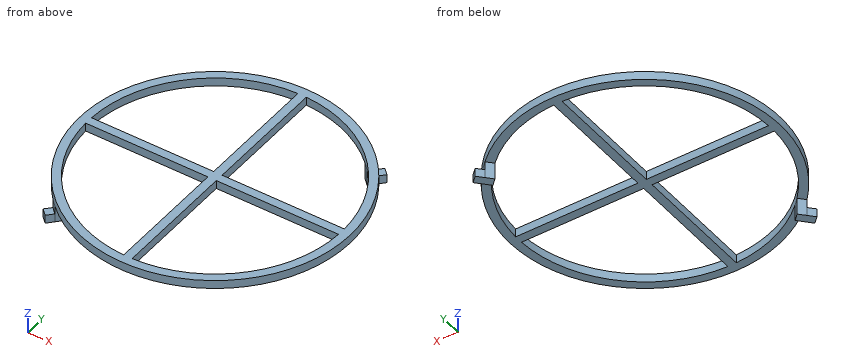
from build123d import *

# Parameters (mm, degrees)
SKETCH1_R           = 16
BOSS_EXTRUDE1_DEPTH = 1
BOSS_EXTRUDE2_DEPTH = 1
BOSS_EXTRUDE3_DEPTH = 1
CIRPATTERN1_COUNT   = 2


with BuildPart() as part:
    # Sketch1 → Boss-Extrude1 (new body)
    with BuildSketch(Plane.XY):
        Circle(SKETCH1_R)
        with BuildLine():
            Line((-0.5, 14.991664351), (-0.5, 0.5))
            Line((-0.5, 0.5), (-14.991664351, 0.5))
            ThreePointArc((-14.991664351, 0.5), (-10.606601718, 10.606601718), (-0.5, 14.991664351))
        make_face(mode=Mode.SUBTRACT)
        with BuildLine():
            Line((0.5, 14.991664351), (0.5, 0.5))
            Line((0.5, 0.5), (14.991664351, 0.5))
            ThreePointArc((14.991664351, 0.5), (10.606601718, 10.606601718), (0.5, 14.991664351))
        make_face(mode=Mode.SUBTRACT)
        with BuildLine():
            Line((-14.991664351, -0.5), (-0.5, -0.5))
            Line((-0.5, -0.5), (-0.5, -14.991664351))
            ThreePointArc((-0.5, -14.991664351), (-10.606601718, -10.606601718), (-14.991664351, -0.5))
        make_face(mode=Mode.SUBTRACT)
        with BuildLine():
            Line((0.5, -0.5), (14.991664351, -0.5))
            ThreePointArc((14.991664351, -0.5), (10.606601718, -10.606601718), (0.5, -14.991664351))
            Line((0.5, -14.991664351), (0.5, -0.5))
        make_face(mode=Mode.SUBTRACT)
    extrude(amount=BOSS_EXTRUDE1_DEPTH)

    # Sketch3 → Boss-Extrude2 (add)
    with BuildSketch(Plane(origin=(0, 0, 0), x_dir=(-1, 0, 0), z_dir=(0, 0, -1))):
        with BuildLine():
            Line((-11.661770518, 10.954593027), (-10.97567443, 10.224214923))
            ThreePointArc((-10.97567443, 10.224214923), (-10.628744174, 10.58441294), (-10.269999326, 10.932845642))
            Line((-10.269999326, 10.932845642), (-10.954665948, 11.661702018))
            ThreePointArc((-10.954665948, 11.661702018), (-11.313743872, 11.313673126), (-11.661770518, 10.954593027))
        make_face()
    boss_extrude2 = extrude(amount=BOSS_EXTRUDE2_DEPTH)

    # Sketch4 → Boss-Extrude3 (add)
    with BuildSketch(Plane(origin=(0, 0, -1), x_dir=(-1, 0, 0), z_dir=(0, 0, -1))):
        with BuildLine():
            Line((-11.661770518, 10.954593027), (-10.97567443, 10.224214923))
            ThreePointArc((-10.97567443, 10.224214923), (-10.628744174, 10.58441294), (-10.269999326, 10.932845642))
            Line((-10.269999326, 10.932845642), (-10.954665948, 11.661702018))
            Line((-10.954665948, 11.661702018), (-11.617936738, 12.367781633))
            Line((-11.617936738, 12.367781633), (-12.34643714, 11.683449403))
            Line((-12.34643714, 11.683449403), (-11.661770518, 10.954593027))
        make_face()
    boss_extrude3 = extrude(amount=BOSS_EXTRUDE3_DEPTH)

    # CirPattern1: Boss-Extrude2, Boss-Extrude3 ×2 about axis
    cirpattern1_axis = Axis((0, 0, 0), (0, 0, 1))
    for i in range(1, CIRPATTERN1_COUNT):
        add(boss_extrude2.rotate(cirpattern1_axis, i * 360 / CIRPATTERN1_COUNT))
        add(boss_extrude3.rotate(cirpattern1_axis, i * 360 / CIRPATTERN1_COUNT))


solid = part.part
Here's how the part is built. I have some questions about the finished solid (model axes, mm). Round coordinates to 2 decimals unless told otherwise and drop trailing zeros. Loops run counter-clockwise (first coordinate to the right, second up) from the corner with the lowest first, then second, coordinate; pieces in that order, holes last. Notation, with made-up numbers: (-4, 51.5) - (11, 51.5) arc R23 cw to (11, 74.5) - close; hole circle Ø11 at (84, -40). An arc over 180 degrees is marked (long way). One line per question, with ' | ' between items. Start each with the question number.
Q1. I want a section at C-C (y = -2). Write out the boundary of the cut face in (x, z), then the cut area to 3 significant figures.
Q2. Please list where these lines run through material, in increasing order: line 1 (X direction, y = -10, z = 0.35); line 2 (Y direction, x = -8, z = 0.7); line 3 (Y direction, x = 5, z = 0.95). Write a range as [from, to].
Q3. I want a section at A-A (z = 0.5). Write out the boundary of the cut face in (x, y), then the cut area to 3 significant figures.
Q4. Will these pins go through, and if not, where does the flat tip stop? pin 1 (0.5 mm diameter, centred on y = 10, z = 0.5, fed in from -X); pin 2 (10 mm diameter, centred on x = 4, y = 11.5, fed in from -Z); pin 3 (2 mm diameter, centred on x = 9, y = 9.5, fed in from +Z) (3 decimals); pin 4 (0.5 mm diameter, centred on y = -5, z = 0.5, fed in from -X).
Q5. I want a section at B-B (x = -6.5). Write out the boundary of the cut face in (y, z).
Response values:
1) outline: (-15.87, 0) - (-14.87, 0) - (-14.87, 1) - (-15.87, 1) - close; (-0.5, 0) - (0.5, 0) - (0.5, 1) - (-0.5, 1) - close; (14.87, 0) - (15.87, 0) - (15.87, 1) - (14.87, 1) - close | area: 3.02 mm²
2) line 1: x = [-12.49, -11.18], [-0.5, 0.5], [11.18, 12.49] | line 2: y = [-13.86, -12.69], [-0.5, 0.5], [12.69, 13.86] | line 3: y = [-15.2, -14.14], [-0.5, 0.5], [14.14, 15.2]
3) outline: circle Ø32 at (0, 0); hole (-14.99, -0.5) arc R15 ccw to (-0.5, -14.99) - (-0.5, -0.5) - close; hole (-14.99, 0.5) - (-0.5, 0.5) - (-0.5, 14.99) arc R15 ccw to start; hole (0.5, -14.99) arc R15 ccw to (14.99, -0.5) - (0.5, -0.5) - close; hole (0.5, 0.5) - (14.99, 0.5) arc R15 ccw to (0.5, 14.99) - close | area: 156 mm²
4) pin 1: stops at x = -12.69 | pin 2: stops at z = 0 | pin 3: passes through | pin 4: stops at x = -15.28
5) outline: (-14.62, 0) - (-13.52, 0) - (-13.52, 1) - (-14.62, 1) - close; (-0.5, 0) - (0.5, 0) - (0.5, 1) - (-0.5, 1) - close; (13.52, 0) - (14.62, 0) - (14.62, 1) - (13.52, 1) - close
